Work out the finished part from the listing and answer in its coordinate system (mm). A direction names the side the tool comes from. Coordinates: 2 decimals unless noted, no trailing zeros. Loops run counter-clockwise (first coordinate to the right, second up) from the corner with the lowest first, then second, coordinate; pieces in that order, holes last.
```python
from build123d import *

# Parameters (mm, degrees)
SKETCH2_W           = 2
SKETCH2_H           = 0.6
BOSS_EXTRUDE1_DEPTH = 6


with BuildPart() as part:
    # Sketch1 → Revolve1 (revolve)
    with BuildSketch(Plane.XY):
        with BuildLine():
            Line((-4.5, 6.6), (-4.5, 2.3))
            Line((-4.5, 2.3), (-6, 2.3))
            Line((-6, 2.3), (-7.25, 1))
            Line((-7.25, 1), (-7.25, 0))
            Line((-7.25, 0), (-6.15, 0))
            Line((-6.15, 0), (-6.15, -10))
            Line((-6.15, -10), (-5.8, -10))
            Line((-5.8, -10), (-5.8, -18))
            Line((-5.8, -18), (0, -18))
            Line((0, -18), (0, 7.1))
            ThreePointArc((0, 7.1), (-2.263846285, 6.974616561), (-4.5, 6.6))
        make_face()
    revolve(axis=Axis((0, 17.963306775, 0), (0, -1, 0)))

    # Sketch2 → Boss-Extrude1 (add)
    with BuildSketch(Plane.XZ.offset(18)):
        with Locations((1, 3)):
            Rectangle(SKETCH2_W, SKETCH2_H)
        with Locations((1, -3)):
            Rectangle(SKETCH2_W, SKETCH2_H)
    extrude(amount=BOSS_EXTRUDE1_DEPTH)


solid = part.part
```
1. Each of these flat-tipped pins is pushed along its axis until it touches: P1, Ø1.6, axis at x = 0.5, y = -20.5, coming from the +Z side; P2, Ø8, axis at y = -5.5, z = 1, coming from the -X side; P3, Ø3.5, axis at x = 2, z = -1, coming from the +Y side. Where does it stop, or does it pass through?
2. A cutting plane is placed at C-C, the plane y = 0.5. Give the vertices of the cut face in (x, z), then the cut area to 3 significant figures.
3. A cutting plane is placed at A-A, the plane y = -19. Give the vertices of the cut face in (x, z), then the cut area to 3 significant figures.
4. Straight lines are drawn through the part: probe 1 along Z at (x, y) = (0, -8); probe 2 along Y at (x, z) = (4.75, -2.25). For each, find the intervals that lie inside material, in ascending order.
5. For faces 1 (the flat face through (1, -21, 3.3)), 2 (the flat face through (2, 0, 6)), 3 (the cylindrical face through (0.59, 4.42, -4.46)), determine the directions among +Z, -Z, +X, -X, +Y, -Y from which every point of the face is accessible in a straight line to the end or side of a thin tool.
6. Determine the mould class of faces 4 (the flat face through (1, -21, -2.7)), 5 (the flat face through (-1.4, 2.3, -4.5)), 6 (the cylindrical face through (5.794, -14.056, -0.255)), 7 (the flat face through (1, -21, -3.3)) for opening direction Z: released by +Z, released by -Z, zero draft, split by the parting line, or undercut.
7. A cutting plane is placed at B-B, the plane z = 0. Give the vertices of the cut face in (x, y).
Answers below:
1. P1: stops at z = 3.3
1. P2: stops at x = -6.15
1. P3: stops at y = 7.09
2. outline: circle Ø14.5 at (0, 0)
2. area: 165 mm2
3. outline: (0, -3.3) - (2, -3.3) - (2, -2.7) - (0, -2.7) - close; (0, 2.7) - (2, 2.7) - (2, 3.3) - (0, 3.3) - close
3. area: 2.40 mm2
4. probe 1: z = -6.15 to 6.15
4. probe 2: y = -18 to 2.3
5. face 1: +Z, +X, -X, -Y
5. face 2: -Y
5. face 3: +Y
6. face 4: undercut
6. face 5: zero draft
6. face 6: split by the parting line
6. face 7: released by -Z
7. outline: (-7.25, 0) - (-6.15, 0) - (-6.15, -10) - (-5.8, -10) - (-5.8, -18) - (5.8, -18) - (5.8, -10) - (6.15, -10) - (6.15, 0) - (7.25, 0) - (7.25, 1) - (6, 2.3) - (4.5, 2.3) - (4.5, 6.6) arc R20.5 ccw to (-4.5, 6.6) - (-4.5, 2.3) - (-6, 2.3) - (-7.25, 1) - close
